Autodesk Inventor part; units mm, degrees
ref_plane "YZ Plane" through (0, 0, 0) normal (1, 0, 0) x (0, 1, 0)
ref_plane "XZ Plane" through (0, 0, 0) normal (0, 1, 0) x (-1, 0, 0)
ref_plane "XY Plane" through (0, 0, 0) normal (0, 0, 1) x (1, 0, 0)
sketch "Sketch1" plane through (0, 0, 0) normal (0, 1, 0) x (-1, 0, 0)
  line L0 (10, 25) -> (-10, 25)
  line L1 (-10, 25) -> (-10, -25)
  line L2 (-10, -25) -> (10, -25)
  line L3 (10, -25) -> (10, 25)
  point P0 (0, 0)
  dimension "d0" = 50
  dimension "d1" = 20
  dimension "d2" = 25
  dimension "d3" = 10
extrude "Extrusion1" add sketch "Sketch1" along normal blind 5
sketch "Sketch2" plane through (0, 5, 0) normal (0, 1, 0) x (1, 0, 0)
  line L0 (-10, -25) -> (10, -25)
  line L1 (-7.5, -25) -> (7.5, -25)
  line L2 (7.5, -25) -> (7.5, -20)
  line L3 (7.5, -20) -> (-7.5, -20)
  line L4 (-7.5, -20) -> (-7.5, -25)
  line L5 (-10, 25) -> (-10, -25)
  line L6 (10, 25) -> (-10, 25)
  line L7 (-7.5, 25) -> (7.5, 25)
  line L8 (7.5, 25) -> (7.5, 20)
  line L9 (7.5, 20) -> (-7.5, 20)
  line L10 (-7.5, 20) -> (-7.5, 25)
  point P0 (0, 0)
  dimension "d6" = 15
  dimension "d7" = 5
  dimension "d8" = 2.5
  dimension "d9" = 5
extrude "Extrusion2" add sketch "Sketch2" along normal blind 50
fillet "Fillet1" radius 5 4 edges at (7.5, 55, 22.5) (7.5, 55, -22.5) (-7.5, 55, 22.5) (-7.5, 55, -22.5)
sketch "Sketch3" plane through (-10, 0, 25) normal (0, 0, 1) x (1, 0, 0)
  line L0 (7.5, 55) -> (12.5, 55)
  circle A0 centre (10, 47) radius 3
  point P0 (10, 0)
  point P1 (10, 55)
  dimension "d13" = 6
  dimension "d14" = 8
extrude "Extrusion3" cut sketch "Sketch3" against normal through all
sketch "Sketch4" plane through (0, 5, 0) normal (0, 1, 0) x (1, 0, 0)
  line L0 (2.5, -20) -> (-2.5, -20)
  line L1 (-2.5, 20) -> (2.5, 20)
  circle A0 centre (0, -14.0028) radius 3
  circle A1 centre (0, 14) radius 3
  point P0 (0, 0)
  point P1 (0, -20)
  dimension "d17" = 6
  dimension "d18" = 6
  dimension "d19" = 5.9972
  dimension "d20" = 6
extrude "Extrusion4" cut sketch "Sketch4" against normal blind 10
properties part number "sensor_cover_ultrasonic_3"
Check sheet for the modelled part. Datum: model origin and axes. Units: mm. A direction names the side the tool comes from. Give positions to 0.01 mm unless a question says otherwise; leave off trailing zeros. Order: outer loops, then holes, each group sorted by start corner. A loop starts at its lowest first (then second) coordinate and runs counter-clockwise, first axis right, second up. Notation, with made-up numbers: M 77.5,44 L 126.5,44 A32 cw 126.5,70 Z; hole C 23,79.25 d1. An arc over 180 degrees is marked long. Answer in a Markdown table with one row per item. Add a question column.
Q1. Sectioned sample at C-C, the plane x = 0. Record the boundary of the cut face in (y, z), and give its area (3 significant figures).
Q2. Access from +Z, -Z, +X, -X, +Y, -Y to the whole of each face (thin tool, end or side, straight path). Record for faces 1 (the flat face through (0, 30, -20)), 2 (the flat face through (7.5, 27, 23)), 3 (the flat face through (-7.5, 27, -22)).
Q3. Sectioned sample at B-B, the plane z = -14. Record the boundary of the cut face in (x, y), and give its area (3 significant figures).
Q4. Sectioned sample at D-D, the plane y = 47. Record the boundary of the cut face in (x, z), and give its area (3 significant figures).
Q5. Release check for a two-part mould opening along Z. For faces 4 (the flat face through (-10, 2, 0)), 5 (the flat face through (0, 27, 25)), 6 (the flat face through (0, 30, 20)) record: released by +Z, released by -Z, zero draft, split by the parting line, or undercut.
Q6. Gauge pin test, flat ends, axial feed: pin 1 Ø3 at (x, z) = (8, 0.5) entering from +Y; pin 2 Ø1.5 at (y, z) = (36.5, 22.5) entering from -X; pin 3 Ø5.5 at (x, y) = (0, 47) entering from +Z; pin 4 Ø1.5 at (y, z) = (22.5, 21.5) entering from +X. Record the tip position at first contact, or that the pin passes through.
Q7. Thickness scan on L1, parallel to Z at x = 0, y = 2.95; L2, parallel to Z at x = 2, y = 29.5; L3, parallel to Y at x = 0, z = -21.35. Record the ranges inside material, lowest first.
Q8. Sectioned sample at A-A, the plane y = 39. Record the boundary of the cut face in (x, z).
Verdict:
| question | item | result |
|---|---|---|
| 1 | outline | M 0,-25 L 44,-25 L 44,-20 L 5,-20 L 5,-17 L 0,-17 Z; M 0,-11 L 5,-11 L 5,11 L 0,11 Z; M 0,17 L 5,17 L 5,20 L 44,20 L 44,25 L 0,25 Z; M 50,-25 L 55,-25 L 55,-20 L 50,-20 Z; M 50,20 L 55,20 L 55,25 L 50,25 Z |
| 1 | area | 630 mm² |
| 2 | face 1 | +X, -X, +Y |
| 2 | face 2 | +Z, -Z, +X, +Y |
| 2 | face 3 | +Z, -Z, -X, +Y |
| 3 | outline | M -10,0 L -3,0 L -3,5 L -10,5 Z; M 3,0 L 10,0 L 10,5 L 3,5 Z |
| 3 | area | 70.0 mm² |
| 4 | outline | M -7.5,-25 L -3,-25 L -3,-20 L -7.5,-20 Z; M -7.5,20 L -3,20 L -3,25 L -7.5,25 Z; M 3,-25 L 7.5,-25 L 7.5,-20 L 3,-20 Z; M 3,20 L 7.5,20 L 7.5,25 L 3,25 Z |
| 4 | area | 90.0 mm² |
| 5 | face 4 | zero draft |
| 5 | face 5 | released by +Z |
| 5 | face 6 | undercut |
| 6 | pin 1 | y = 5 |
| 6 | pin 2 | x = -7.5 |
| 6 | pin 3 | through |
| 6 | pin 4 | x = 7.5 |
| 7 | L1 | -25 to -17, -11 to 11, 17 to 25 |
| 7 | L2 | -25 to -20, 20 to 25 |
| 7 | L3 | 0 to 44, 50 to 55 |
| 8 | outline | M -7.5,-25 L 7.5,-25 L 7.5,-20 L -7.5,-20 Z; M -7.5,20 L 7.5,20 L 7.5,25 L -7.5,25 Z |
